```python
from build123d import *

# Parameters (mm, degrees)
F0_W         = 5.3462936
F0_H         = 14.732
F0_W_2       = 5.5306468
F0_H_2       = 12.7
F1_DEPTH     = 6.35
F2_T1_DEPTH  = 27.432
F2_T3_DEPTH  = 40.132
F2_T6_ANGLE  = 180
F2_T8_ANGLE  = 180
F2_T10_ANGLE = 180
F2_T12_ANGLE = 180


# Not quite as in the source:
# - a fillet or chamfer that OpenCascade refuses, or shapes differently, is made with other operations: its cross-section is extruded or revolved along the edge and cut away or added


with BuildPart() as f1:
    # F0 (on Front) → F1 (new body)
    with BuildSketch(Plane.XZ):
        with BuildLine():
            Line((-2.9891021488, 14.732), (-2.9891021488, 0))
            Line((-2.9891021488, 0), (2.5415446512, 0))
            Line((2.5415446512, 0), (2.5415446512, 14.732))
            ThreePointArc((2.5415446512, 14.732), (8.0721914512, 20.2626468), (13.6028382512, 14.732))
            Line((13.6028382512, 14.732), (18.9491318512, 14.732))
            ThreePointArc((18.9491318512, 14.732), (7.9800148512, 25.701117), (-2.9891021488, 14.732))
        make_face()
        with Locations((16.2759850512, 7.366)):
            Rectangle(F0_W, F0_H)
        with Locations((-0.2237787488, -6.35)):
            Rectangle(F0_W_2, F0_H_2)
    extrude(amount=F1_DEPTH)

    # F2: fillet of radius 5.08 on 4 edges, made by hand

    # F2_s2 → F2_t1 (cut)
    with BuildSketch(Plane.XY.offset(-12.7)):
        with BuildLine():
            ThreePointArc((18.9491318512, -5.08), (17.4612342996, -1.4878975516), (13.8691318512, 0))
            Line((13.8691318512, 0), (18.9491318512, 0))
            Line((18.9491318512, 0), (18.9491318512, -5.08))
        make_face()
        with BuildLine():
            ThreePointArc((13.6028382512, -5.08), (15.0907358028, -1.4878975516), (18.6828382512, 0))
            Line((18.6828382512, 0), (13.6028382512, 0))
            Line((13.6028382512, 0), (13.6028382512, -5.08))
        make_face()
        with BuildLine():
            ThreePointArc((13.6028382512, -1.27), (15.0907358028, -4.8621024484), (18.6828382512, -6.35))
            Line((18.6828382512, -6.35), (13.6028382512, -6.35))
            Line((13.6028382512, -6.35), (13.6028382512, -1.27))
        make_face()
        with BuildLine():
            ThreePointArc((18.9491318512, -1.27), (17.4612342996, -4.8621024484), (13.8691318512, -6.35))
            Line((13.8691318512, -6.35), (18.9491318512, -6.35))
            Line((18.9491318512, -6.35), (18.9491318512, -1.27))
        make_face()
    extrude(amount=F2_T1_DEPTH, mode=Mode.SUBTRACT)

    # F2_s4 → F2_t3 (cut)
    with BuildSketch(Plane.XY.offset(-25.4)):
        with BuildLine():
            ThreePointArc((2.5415446512, -1.27), (1.0536470996, -4.8621024484), (-2.5384553488, -6.35))
            Line((-2.5384553488, -6.35), (2.5415446512, -6.35))
            Line((2.5415446512, -6.35), (2.5415446512, -1.27))
        make_face()
        with BuildLine():
            ThreePointArc((2.5415446512, -5.08), (1.0536470996, -1.4878975516), (-2.5384553488, 0))
            Line((-2.5384553488, 0), (2.5415446512, 0))
            Line((2.5415446512, 0), (2.5415446512, -5.08))
        make_face()
        with BuildLine():
            ThreePointArc((-2.9891021488, -5.08), (-1.5012045972, -1.4878975516), (2.0908978512, 0))
            Line((2.0908978512, 0), (-2.9891021488, 0))
            Line((-2.9891021488, 0), (-2.9891021488, -5.08))
        make_face()
        with BuildLine():
            ThreePointArc((-2.9891021488, -1.27), (-1.5012045972, -4.8621024484), (2.0908978512, -6.35))
            Line((2.0908978512, -6.35), (-2.9891021488, -6.35))
            Line((-2.9891021488, -6.35), (-2.9891021488, -1.27))
        make_face()
    extrude(amount=F2_T3_DEPTH, mode=Mode.SUBTRACT)

    # F2_s5 → F2_t6 (revolve, cut)
    with BuildSketch(Plane.XY.offset(14.732)):
        with BuildLine():
            ThreePointArc((18.9491318512, -1.27), (17.4612342996, -4.8621024484), (13.8691318512, -6.35))
            Line((13.8691318512, -6.35), (18.9491318512, -6.35))
            Line((18.9491318512, -6.35), (18.9491318512, -1.27))
        make_face()
    revolve(axis=Axis((7.9800148512, -6.35, 14.732), (0, -1, 0)), revolution_arc=F2_T6_ANGLE, mode=Mode.SUBTRACT)

    # F2_s7 → F2_t8 (revolve, cut)
    with BuildSketch(Plane.XY.offset(14.732)):
        with BuildLine():
            ThreePointArc((2.5415446512, -5.08), (1.0536470996, -1.4878975516), (-2.5384553488, 0))
            Line((-2.5384553488, 0), (2.5415446512, 0))
            Line((2.5415446512, 0), (2.5415446512, -5.08))
        make_face()
    revolve(axis=Axis((8.0721914512, 0, 14.732), (0, 1, 0)), revolution_arc=F2_T8_ANGLE, mode=Mode.SUBTRACT)

    # F2_s9 → F2_t10 (revolve, cut)
    with BuildSketch(Plane.XY.offset(14.732)):
        with BuildLine():
            ThreePointArc((2.5415446512, -1.27), (1.0536470996, -4.8621024484), (-2.5384553488, -6.35))
            Line((-2.5384553488, -6.35), (2.5415446512, -6.35))
            Line((2.5415446512, -6.35), (2.5415446512, -1.27))
        make_face()
    revolve(axis=Axis((8.0721914512, -6.35, 14.732), (0, 1, 0)), revolution_arc=F2_T10_ANGLE, mode=Mode.SUBTRACT)

    # F2_s11 → F2_t12 (revolve, cut)
    with BuildSketch(Plane.XY.offset(14.732)):
        with BuildLine():
            ThreePointArc((18.9491318512, -5.08), (17.4612342996, -1.4878975516), (13.8691318512, 0))
            Line((13.8691318512, 0), (18.9491318512, 0))
            Line((18.9491318512, 0), (18.9491318512, -5.08))
        make_face()
    revolve(axis=Axis((7.9800148512, 0, 14.732), (0, -1, 0)), revolution_arc=F2_T12_ANGLE, mode=Mode.SUBTRACT)


solid = f1.part
```
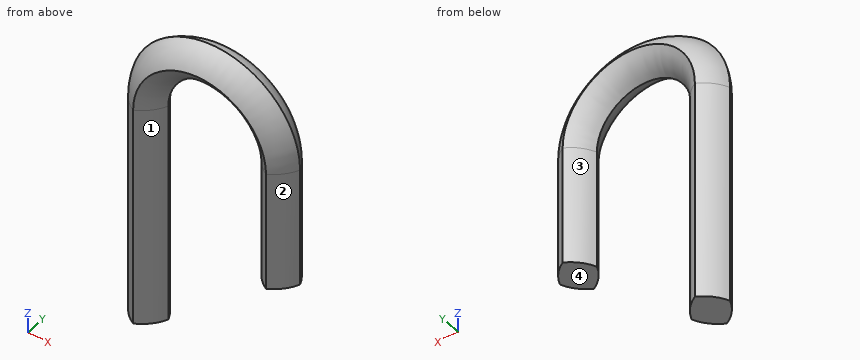
Read the model definition and answer for the solid it produces. Units are mm, in the model's axes. Face numbers are marked on the shaded views. Coordinates: 2 decimals unless noted, no trailing zeros. Loops run counter-clockwise (first coordinate to the right, second up) from the corner with the lowest first, then second, coordinate; pieces in that order, holes last.
(1) Flat-ended cylindrical pins translate along their axes: pin 1 Ø2 at (x, z) = (13, 19) entering from +Y; pin 2 Ø1 at (x, z) = (16, 21) entering from -Y; pin 3 Ø1.4 at (x, y) = (16.5, -2) entering from -Z. Find the tip coordinate at first contact, or state that the pin passes through.
Solution:
pin 1: stops at y = -1.05
pin 2: stops at y = -4.65
pin 3: stops at z = 0
(2) The part is cut by section A-A (z = 6.5). Determine the outline of the cut face in (x, y) (3 decimals), and give its area (3 significant figures).
Solution:
outline: (-2.618, -3.175) arc R5.08 ccw to (-0.224, -5.792) arc R5.08 ccw to (2.171, -3.175) arc R5.08 ccw to (-0.224, -0.558) arc R5.08 ccw to start; (13.974, -3.175) arc R5.08 ccw to (16.276, -5.744) arc R5.08 ccw to (18.578, -3.175) arc R5.08 ccw to (16.276, -0.606) arc R5.08 ccw to start
area: 30.2 mm2
(3) The part is cut by section C-C (z = -7). Determine the outline of the cut face in (x, y) (3 decimals), and give its area (3 significant figures).
Solution:
outline: (-2.618, -3.175) arc R5.08 ccw to (-0.224, -5.792) arc R5.08 ccw to (2.171, -3.175) arc R5.08 ccw to (-0.224, -0.558) arc R5.08 ccw to start
area: 15.6 mm2
(4) Consider line 1 along X through (y, z) = (-3.4, 16); line 2 along X through (y, z) = (-3.65, 7.5); line 3 along Y through (x, z) = (4.25, 22). Determine where each line is inside the solid, lowest interval first.
Solution:
line 1: x = -2.44 to 2.21, 13.94 to 18.4
line 2: x = -2.4 to 1.95, 14.19 to 18.36
line 3: y = -5.75 to -0.6
(5) The mould has two halves that part along X. Classify the marked faces 1, 2, 3 and 4: released by +X, released by -X, zero draft, split by the parting line, or undercut.
Solution:
face 1: undercut
face 2: released by +X
face 3: undercut
face 4: zero draft
(6) The part is cut by section B-B (y = -3.9). Determine the outline of the cut face in (x, z), and give its area (3 significant figures).
Solution:
outline: (-2.26, -12.7) - (1.81, -12.7) - (1.81, 14.73) arc R6.26 cw to (14.34, 14.73) - (14.34, 0) - (18.22, 0) - (18.22, 14.73) arc R10.24 ccw to (-2.26, 14.73) - close
area: 272 mm2
